Autodesk Inventor part; units mm, degrees
ref_plane "YZ Plane" through (0, 0, 0) normal (1, 0, 0) x (0, 1, 0)
ref_plane "XZ Plane" through (0, 0, 0) normal (0, 1, 0) x (-1, 0, 0)
ref_plane "XY Plane" through (0, 0, 0) normal (0, 0, 1) x (1, 0, 0)
sketch "Sketch1" plane through (0, 0, 0) normal (1, 0, 0) x (0, 1, 0)
  line L0 (-5.8, 12.5) -> (-15, 12.5)
  line L1 (-5.8, -12.5) -> (-15, -12.5)
  line L2 (-5.8, 12.5) -> (8.6392, 7.25)
  line L3 (-5.8, -12.5) -> (8.6392, -7.25)
  arc A0 (8.6392, -7.25) -> (8.6392, 7.25) centre (5.5639, 0) ccw
  line L4 (-15, 12.5) -> (-15, 18.5)
  line L5 (-15, 18.5) -> (23.4392, 18.5)
  line L6 (23.4392, 18.5) -> (23.4392, -18.5)
  line L7 (23.4392, -18.5) -> (-15, -18.5)
  line L8 (-15, -18.5) -> (-15, -12.5)
  line L9 (23.4392, 0) -> (13.4392, 0) construction
  line L10 (13.4392, 0) -> (0, 0) construction
  line L11 (8.6392, -7.25) -> (8.6392, 0) construction
  line L12 (8.6392, 0) -> (8.6392, 7.25) construction
  point P0 (-10.4, 12.5)
  dimension "d0" = 9.2
  dimension "d1" = 25
  dimension "d2" = 12.5
  dimension "d7" = 9.2
  dimension "d8" = 12.5
  dimension "d9" = 15
  dimension "d10" = 15
  dimension "d14" = 6
  dimension "d15" = 6
  dimension "d16" = 37
  dimension "d29" = 10
  dimension "d88" = 4.8
  dimension "d90" = 14.5
  dimension "d91" = 23.4392
extrude "Extrusion1" add sketch "Sketch1" along normal blind 20
sketch "Sketch2" plane through (0, 23.4392, 18.5) normal (0, 1, 0) x (1, 0, 0)
  line L0 (0, 31) -> (0, 37)
  line L1 (0, 37) -> (70, 37)
  line L2 (70, 37) -> (70, 0.0995)
  line L3 (70, 0.0995) -> (0, 0.0995)
  line L4 (0, 0.0995) -> (0, 37)
  line L5 (20, 37) -> (20, 0)
  point P0 (0, 18.5)
  point P1 (70, 18.5498)
  dimension "d19" = 50
extrude "Extrusion2" add sketch "Sketch2" along normal blind 10
sketch "Sketch3" plane through (0, 23.4392, 18.5) normal (0, -1, 0) x (1, 0, 0)
  line L0 (110.5, -8.5498) -> (110.5, -28.5498)
  line L1 (110.5, -28.5498) -> (70, -28.5498)
  line L2 (70, -28.5498) -> (70, -8.5498)
  line L3 (70, -0.0995) -> (70, -37)
  line L4 (110.5, -8.5498) -> (119.5, -8.5498)
  line L5 (119.5, -8.5498) -> (119.5, -37)
  line L6 (119.5, -37) -> (70, -37)
  line L7 (70, -37) -> (0, -37)
  line L8 (70, -37) -> (59, -37)
  line L9 (59, -37) -> (59, -8.5498)
  line L10 (59, -8.5498) -> (70, -8.5498)
  point P0 (0, -18.5)
  point P1 (70, -18.5498)
  point P2 (70, -18.5498)
  point P3 (110.5, -18.5498)
  dimension "d22" = 20
  dimension "d23" = 20
  dimension "d24" = 0
  dimension "d25" = 40.5
  dimension "d26" = 9
  dimension "d30" = 11
extrude "Extrusion3" add sketch "Sketch3" along normal blind 9.5 and the other way blind 10
sketch "Sketch4" plane through (0, 33.4392, 18.5) normal (0, 1, 0) x (1, 0, 0)
  line L0 (110.5, 8.5498) -> (119.5, 8.5498)
  line L1 (62.5, 28.5653) -> (119.5, 28.5653)
  line L2 (119.5, 28.5653) -> (119.5, 8.5498)
  line L3 (119.5, 8.5498) -> (62.5, 8.5498)
  line L4 (62.5, 8.5498) -> (62.5, 28.5653)
  line L5 (70, 0.0995) -> (70, 28.5498)
  line L6 (110.5, 28.5498) -> (110.5, 8.5498)
  point P0 (0, 18.5)
  point P1 (70, 14.3246)
  point P2 (110.5, 8.5498)
  dimension "d33" = 7.5
  dimension "d34" = 9
extrude "Extrusion4" cut sketch "Sketch4" against normal blind 14.2625
sketch "Sketch5" plane through (0, 33.4392, 18.5) normal (0, 1, 0) x (1, 0, 0)
  line L0 (62.5, 8.5498) -> (62.5, 28.5653)
  line L1 (62.5, 8.5498) -> (70, 8.5498)
  line L2 (70, 8.5498) -> (70, -1.0168)
  line L3 (70, -1.0168) -> (62.5, -1.0168)
  line L4 (62.5, -1.0168) -> (62.5, 8.5498)
  line L5 (70, 0.0995) -> (70, 8.5498)
  point P0 (0, 18.5)
  dimension "d47" = 0
extrude "Extrusion5" cut sketch "Sketch5" against normal blind 14.2625
sketch "Sketch7" plane through (59, 13.9392, 9.9502) normal (0, 0, 1) x (1, 0, 0)
  line L0 (3.5, 5.2375) -> (3.5, 9.5)
  line L1 (11, 0) -> (11, 5.2375)
  line L2 (3.5, 5.2375) -> (11, 5.2375)
  line L3 (11, 5.2375) -> (11, 0)
  line L4 (11, 0) -> (0, 0)
  line L5 (0, 0) -> (0, 9.5)
  line L6 (0, 9.5) -> (3.5, 9.5)
  line L7 (-39, 9.5) -> (3.5, 9.5)
  line L8 (3.5, 9.5) -> (3.5, 19.5)
  point P0 (-59, -13.9392)
  dimension "d42" = 11
  dimension "d43" = 0
  dimension "d44" = 0
extrude "Extrusion7" add sketch "Sketch7" along normal blind 8.45
sketch "Sketch8" plane through (62.5, 33.4392, 18.4005) normal (1, 0, 0) x (0, 0, -1)
  line L0 (28.4658, 0) -> (28.4658, -14.2625)
  line L1 (36.9005, 0) -> (0, 0)
  line L2 (28.4658, -9.8625) -> (0, -9.8625)
  line L3 (0, -9.8625) -> (0, 0)
  line L4 (0, 0) -> (28.4658, 0)
  line L5 (28.4658, 0) -> (28.4658, -9.8625)
  line L6 (28.4658, -14.2625) -> (8.4502, -14.2625)
  line L7 (8.4502, -14.2625) -> (8.4502, -19.5)
  line L8 (0, -10) -> (0, 0)
  point P0 (18.4005, -33.4392)
  dimension "d48" = 4.4
  dimension "d52" = 0
extrude "Extrusion8" add sketch "Sketch8" along normal blind 7.5
sketch "Sketch9" plane through (0, 33.4392, 18.5) normal (0, 1, 0) x (1, 0, 0)
  line L0 (59, 37) -> (59, 0.0998)
  line L1 (59, 0.0998) -> (59, 37)
  line L2 (119.5, 37) -> (119.5, 8.5498)
  line L3 (59, 37) -> (119.5, 37)
  line L4 (70, 28.5653) -> (119.5, 28.5653)
  line L5 (119.5, 37) -> (119.5, 28.5653)
  line L6 (119.5, 28.5653) -> (70, 28.5653)
  line L7 (0, 0.0995) -> (70, 0.0995)
  line L8 (70, 28.5653) -> (70, 0.0995)
  line L9 (70, 0.0995) -> (59, 0.0998)
  point P0 (0, 18.5)
extrude "Extrusion9" add sketch "Sketch9" along normal blind 16
sketch "Sketch10" plane through (0, 33.4392, 18.5) normal (0, 1, 0) x (1, 0, 0)
  line L0 (59, 0.0998) -> (59, 37)
  line L1 (0, 0.0995) -> (70, 0.0995)
  line L2 (59, 37) -> (0, 37)
  line L3 (0, 37) -> (0, 0.0995)
  line L4 (0, 0.0995) -> (59, 0.0995)
  line L5 (59, 0.0995) -> (59, 37)
  point P0 (0, 18.5)
  point P1 (59, 0.0995)
extrude "Extrusion10" add sketch "Sketch10" along normal blind 16
sketch "Sketch12" plane through (0, 49.4392, 18.5) normal (0, 1, 0) x (1, 0, 0)
  line L0 (70, 28.5498) -> (70, 0.0998)
  line L1 (70, 0.0998) -> (-11.6844, 0.0998)
  line L2 (-11.6844, 0.0998) -> (-11.6844, -16.6848)
  line L3 (-11.6844, -16.6848) -> (70, -16.6848)
  line L4 (70, -16.6848) -> (70, 0.0998)
  point P0 (0, 18.5)
extrude "Extrusion11" cut sketch "Sketch12" against normal blind 76.325
sketch "Sketch13" plane through (0, 19.1767, 18.5) normal (0, 1, 0) x (1, 0, 0)
  line L0 (110.5, 8.5498) -> (110.5, 28.5498)
  line L1 (70, 0.0998) -> (70, 28.5653)
  line L2 (110.5, 28.5498) -> (70, 28.5498)
  line L3 (70, 28.5498) -> (70, 28.5653)
  line L4 (70, 28.5653) -> (110.5, 28.5653)
  line L5 (110.5, 28.5653) -> (110.5, 28.5498)
  point P0 (0, 18.5)
extrude "Extrusion12" cut sketch "Sketch13" against normal blind 76.325
sketch "Sketch14" plane through (0, 13.9392, 18.5) normal (0, -1, 0) x (1, 0, 0)
  circle A0 centre (114.7, -23.3) radius 2.1
  circle A1 centre (114.7, -13.2) radius 2.1
  line L0 (110.5, -8.5498) -> (110.5, -28.5653)
  line L1 (20, -11.25) -> (20, -25.75)
  point P0 (0, -18.5)
  point P1 (20, -18.5)
  dimension "d61" = 4.2
  dimension "d62" = 4.2
  dimension "d63" = 10.1
  dimension "d64" = 4.2
  dimension "d65" = 0
  dimension "d66" = 4.8
extrude "Extrusion13" cut sketch "Sketch14" against normal blind 12.825
pattern_linear "Rectangular Pattern1" count 2 spacing 49 along (-1, 0, 0) of "Extrusion13"
sketch "Sketch15" plane through (0, 13.9392, 18.5) normal (0, -1, 0) x (1, 0, 0)
  line L0 (70, -0.0998) -> (70, -28.5653)
  line L1 (70, -0.0998) -> (119.5, -0.0998)
  line L2 (119.5, -0.0998) -> (119.5, -8.5498)
  line L3 (119.5, -8.5498) -> (110.5, -8.5498)
  line L4 (119.5, -8.5498) -> (110.5, -8.5498)
  line L5 (110.5, -8.5498) -> (68.2571, -8.5498)
  line L6 (68.2571, -8.5498) -> (59, -8.5498)
  line L7 (59, -37) -> (59, -0.0998)
  line L8 (59, -0.0998) -> (59, -8.5498)
  line L9 (59, -0.0998) -> (70, -0.0998)
  point P0 (0, -18.5)
extrude "Extrusion14" add sketch "Sketch15" against normal blind 35.5
sketch "Sketch16" plane through (119.5, 13.9392, 18.4002) normal (1, 0, 0) x (0, 0, -1)
  line L0 (7.45, 5.2375) -> (29.4655, 5.2375)
  line L1 (29.4655, 5.2375) -> (29.4655, 38.0522)
  line L2 (29.4655, 38.0522) -> (7.45, 38.0522)
  line L3 (7.45, 38.0522) -> (7.45, 5.2375)
  line L4 (28.4655, 5.2375) -> (8.45, 5.2375)
  line L5 (8.45, 5.2375) -> (8.45, 35.5)
  line L6 (28.4655, 35.5) -> (28.4655, 5.2375)
  point P0 (18.4002, -13.9392)
  dimension "d74" = 0
  dimension "d75" = 1
  dimension "d76" = 1
extrude "Extrusion15" cut sketch "Sketch16" against normal blind 49.6875
sketch "Sketch19" plane through (0, 13.9392, 18.5) normal (0, -1, 0) x (1, 0, 0)
  line L0 (134.9623, 3.6486) -> (95.7961, 3.6486)
  line L1 (95.7961, 3.6486) -> (95.7961, -43.9762)
  line L2 (95.7961, -43.9762) -> (134.9623, -43.9762)
  line L3 (134.9623, -43.9762) -> (134.9623, 3.6486)
  point P0 (0, -18.5)
extrude "Extrusion18" cut sketch "Sketch19" against normal blind 65.5625
sketch "Sketch20" plane through (0, 49.4392, 18.5) normal (0, 1, 0) x (1, 0, 0)
  line L0 (95.7961, 28.5653) -> (95.7961, 29.5653)
  line L1 (95.7961, 7.5498) -> (69.8125, 7.5498)
  line L2 (95.7961, 29.5653) -> (69.8125, 29.5653)
  line L3 (69.8125, 29.5653) -> (69.8125, 7.5498)
  line L4 (69.8125, 7.5498) -> (95.7961, 7.5498)
  line L5 (95.7961, 7.5498) -> (95.7961, 29.5653)
  point P0 (0, 18.5)
  point P1 (95.7961, 7.5498)
extrude "Extrusion19" cut sketch "Sketch20" against normal blind 65.5625
properties part number "Holder223"
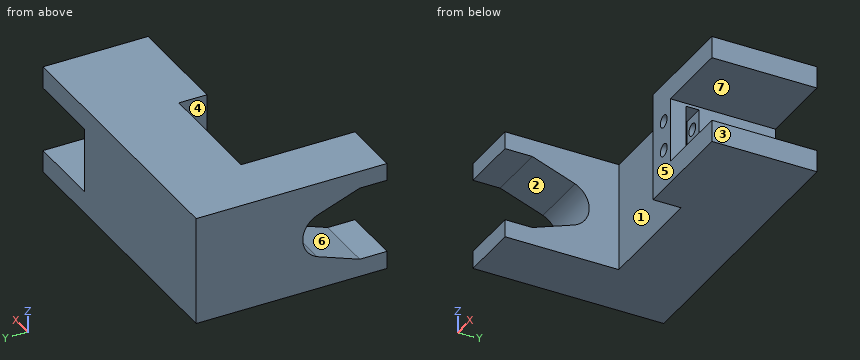
CAD build for the part. Positions are in the model's coordinates, mm. Face numbers are marked on the shaded views. A direction names the side the tool comes from. Round coordinates to 2 decimals unless told otherwise and drop trailing zeros. Loops run counter-clockwise (first coordinate to the right, second up) from the corner with the lowest first, then second, coordinate; pieces in that order, holes last. Notation, with made-up numbers: (-29, 75.25) - (-7, 75.25) arc R32 ccw to (-7, 103.25) - close; hole circle Ø5 at (-20.5, -40). An arc over 180 degrees is marked (long way). Return JSON: item names as keys, results as strings. Group by question number.
Q1. Flat gauge pins, fed straight in: pin 1 Ø8 at (y, z) = (25, -1.5) entering from +X; pin 2 Ø2 at (x, y) = (56.5, 17.5) entering from +Z; pin 3 Ø1.3 at (x, z) = (66.5, -4.5) entering from -Y; pin 4 Ø8 at (x, z) = (64.5, -1.5) entering from -Y. Where does each tip first touch, or does it go through?
Q2. Band-saw the part on C-C on z = 5.3. Give the cut face in (x, y).
Q3. Band-saw the part on D-D on y = 6. Give the cut face in (x, z).
Q4. Tool access for the marked faces 5, 6 and 7: list every direction of +Z, -Z, +X, -X, +Y, -Y with a clear straight run to the whole face (end or side of a thin tool).
Q5. Drill centre lines: line 1 along Z through (x, y) = (65.7, 16); line 2 along Z through (x, y) = (73, 38); line 3 along X through (y, z) = (20, -7). Where is each one in solid material? Low to high. Write a range as [from, to].
Q6. Two-plate mould, pull along X, no slides. Class the marked faces 1, 2, 3 and 4: +X half, -X half, draft (parallel to the pull), parting line (faces both ways), or undercut.
Q7. Band-saw the part on B-B on x = 65.7. Give the cut face in (y, z), plus the area to 3 significant figures.
Q8. Band-saw the part on A-A on y = 17.5. Give the cut face in (x, z), plus the area to 3 significant figures.
Solutions:
{
 "1": {"pin 1": "stops at x = 69.81", "pin 2": "passes through", "pin 3": "stops at y = 26.76", "pin 4": "stops at y = 13.94"},
 "2": {"outline": "(0, 11.39) - (20, 11.39) - (20, 23.44) - (59, 23.44) - (59, 13.94) - (63.6, 13.94) - (63.6, 19.18) - (62.5, 19.18) - (62.5, 23.58) - (63.6, 23.58) - (63.6, 26.76) - (67.8, 26.76) - (67.8, 23.58) - (69.81, 23.58) - (69.81, 49.44) - (0, 49.44) - close; (67.8, 13.94) - (69.81, 13.94) - (69.81, 19.18) - (67.8, 19.18) - close"},
 "3": {"outline": "(0, -18.5) - (20, -18.5) - (20, -8.21) - (0, -8.21) - close; (0, 8.21) - (20, 8.21) - (20, 18.4) - (0, 18.4) - close"},
 "4": {"face 5": "+Z, -Z, +X, -Y", "face 6": "+X, -X, -Y", "face 7": "+X, +Y, -Y"},
 "5": {"line 1": "z = [-18.5, -6.9], [-2.7, 3.2], [7.4, 18.4]", "line 2": "z = [-18.5, -11.07], [10.95, 18.4]", "line 3": "x = [0, 20], [59, 62.5]"},
 "6": {"face 1": "undercut", "face 2": "draft", "face 3": "+X half", "face 4": "undercut"},
 "7": {"outline": "(13.94, -18.5) - (49.44, -18.5) - (49.44, 18.4) - (13.94, 18.4) - (13.94, 7.4) - (19.18, 7.4) - (19.18, 9.95) - (23.58, 9.95) - (23.58, 7.4) - (26.76, 7.4) - (26.76, 3.2) - (23.58, 3.2) - (23.58, -2.7) - (26.76, -2.7) - (26.76, -6.9) - (23.58, -6.9) - (23.58, -10.07) - (19.18, -10.07) - (19.18, -6.9) - (13.94, -6.9) - close; (13.94, -2.7) - (19.18, -2.7) - (19.18, 3.2) - (13.94, 3.2) - close", "area": "1,150 mm^2"},
 "8": {"outline": "(0, -18.5) - (20, -18.5) - (20, 18.4) - (0, 18.4) - close; (59, -18.5) - (95.8, -18.5) - (95.8, -11.07) - (69.81, -11.07) - (69.81, 10.95) - (95.8, 10.95) - (95.8, 18.4) - (59, 18.4) - close; hole circle Ø4.2 at (65.7, -4.8); hole circle Ø4.2 at (65.7, 5.3)", "area": "1,500 mm^2"}
}
